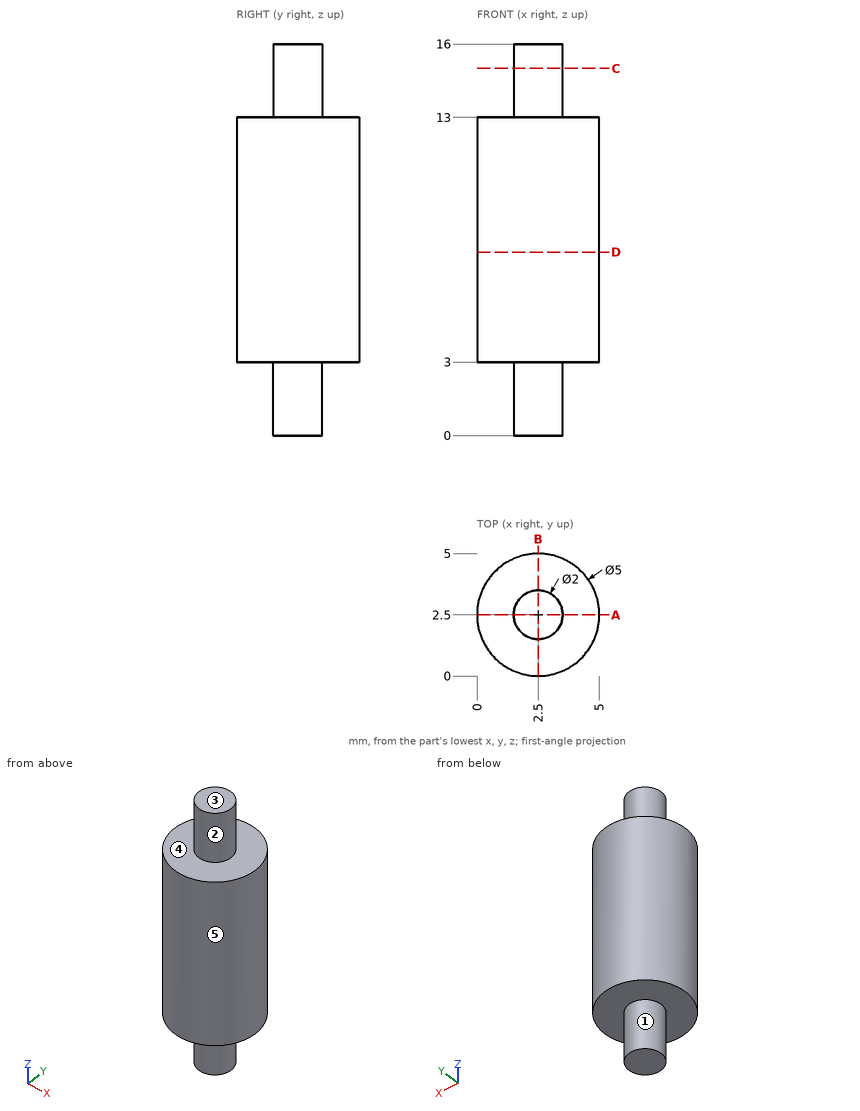
Job drawing, mm, ordinate dimensions from the low corner. One solid piece. A direction names the side the tool comes from. Round coordinates to 2 decimals unless told otherwise and drop trailing zeros. Order: outer loops, then holes, each group sorted by start corner. A loop starts at its lowest first (then second) coordinate and runs counter-clockwise, first axis right, second up. Notation, with made-up numbers: (79.25, 34) -> (110.25, 34) arc R30 cw to (110.25, 69) -> close; hole circle Ø6 at (57.25, 20). An arc over 180 degrees is marked (long way). Write item = value, one per line.
(1) Cut at A-A (y = 2.5). Write the cut outline in (x, z).
Answers follow:
outline = (0, 3) -> (1.5, 3) -> (1.5, 0) -> (3.5, 0) -> (3.5, 3) -> (5, 3) -> (5, 13) -> (3.5, 13) -> (3.5, 16) -> (1.5, 16) -> (1.5, 13) -> (0, 13) -> close
(2) Drill centre lines: L1, parallel to Z at x = 1.75, y = 3.85; L2, parallel to Y at x = 2.6, z = 9; L3, parallel to X at y = 1.05, z = 5.75. Where is each one in solid material? Low to high.
Answers follow:
L1 = 3 to 13
L2 = 0 to 5
L3 = 0.46 to 4.54
(3) Cut at C-C (z = 15). Write the cut outline in (x, y), plus the area to 3 significant figures.
Answers follow:
outline = circle Ø2 at (2.5, 2.5)
area = 3.14 mm²
(4) 3-axis set-ups, long thin cutter, end or side, ignore diameter. For the marked faces 1, 2 and 3: which of +Z, -Z, +X, -X, +Y, -Y reach the whole face in a straight line?
Answers follow:
face_1 = -Z
face_2 = +Z
face_3 = +Z, +X, -X, +Y, -Y
(5) Cut at D-D (z = 7.5). Write the cut outline in (x, y), plus the area to 3 significant figures.
Answers follow:
outline = circle Ø5 at (2.5, 2.5)
area = 19.6 mm²
(6) Flat gauge pins, fed straight in: P1, Ø2, axis at x = 1, y = 2.5, coming from the -Z side; P2, Ø2, axis at x = 4, z = 3.5, coming from the -Y side; P3, Ø1.5, axis at y = 3.5, z = 2.5, coming from the -X side. Where does each tip first touch, or does it go through?
Answers follow:
P1 = 0
P2 = 0.05
P3 = 0.04
(7) Pull direction Y, two halves, no side cores. Call the marked faces 4 and 5: +Y half, -Y half, draft (parallel to the pull), parting line (faces both ways), or undercut.
Answers follow:
face_4 = draft
face_5 = parting line
